Part print with two shaded views. Sizes in mm from the minimum x, y, z corner. A direction names the side the tool comes from. Round coordinates to 2 decimals unless told otherwise and drop trailing zeros. Loops run counter-clockwise (first coordinate to the right, second up) from the corner with the lowest first, then second, coordinate; pieces in that order, holes last. Notation, with made-up numbers: (44, -25.5) - (79, -25.5) arc R26 ccw to (79, -5.5) - close; hole circle Ø3 at (31, -8). An arc over 180 degrees is marked (long way). One line per question, with ' | ' between items.
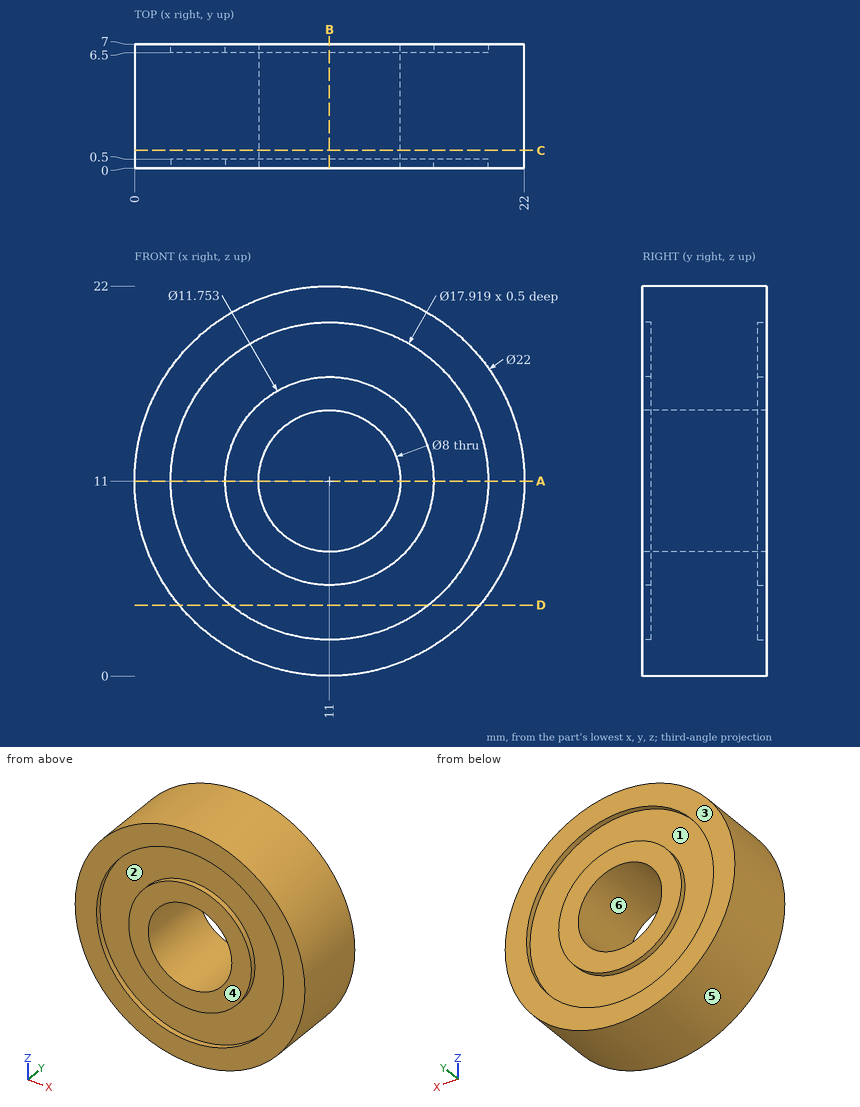
(1) Drop flat-ended pins along their axis: P1, Ø4, axis at x = 18, y = 2, coming from the +Z side; P2, Ø4, axis at x = 8, y = 1, coming from the +Z side; P3, Ø1, axis at y = 5.5, z = 12.5, coming from the -X side. Give the stop position or say it passes through.
Results found:
P1: stops at z = 20.8 | P2: stops at z = 21.95 | P3: stops at x = 0.05
(2) Cut at C-C, the plane y = 1. Write the cut outline in (x, z), then the cut area to 3 significant figures.
Results found:
outline: circle Ø22 at (11, 11); hole circle Ø8 at (11, 11) | area: 330 mm²
(3) Two-plate mould, pull along Z, no slides. Class the marked faces 4, 5 and 6: released by +Z, released by -Z, zero draft, split by the parting line, or undercut.
Results found:
face 4: zero draft | face 5: split by the parting line | face 6: undercut
(4) Probe L1, parallel to X at y = 6.95, z = 11; L2, parallel to X at y = 5.75, z = 11. List the from-to ranges inside material, lowest first.
Results found:
L1: x = 0 to 2.04, 5.12 to 7, 15 to 16.88, 19.96 to 22 | L2: x = 0 to 7, 15 to 22
(5) Cut at B-B, the plane x = 11. Write the cut outline in (y, z).
Results found:
outline: (0, 0) - (7, 0) - (7, 2.04) - (6.5, 2.04) - (6.5, 5.12) - (7, 5.12) - (7, 7) - (0, 7) - (0, 5.12) - (0.5, 5.12) - (0.5, 2.04) - (0, 2.04) - close; (0, 15) - (7, 15) - (7, 16.88) - (6.5, 16.88) - (6.5, 19.96) - (7, 19.96) - (7, 22) - (0, 22) - (0, 19.96) - (0.5, 19.96) - (0.5, 16.88) - (0, 16.88) - close
(6) Tool access for the marked faces 1, 2 and 3: list every direction of +Z, -Z, +X, -X, +Y, -Y with a clear straight run to the whole face (end or side of a thin tool).
Results found:
face 1: +Y | face 2: -Y | face 3: +Z, -Z, +X, -X, +Y
(7) Cut at A-A, the plane z = 11. Write the cut outline in (x, y).
Results found:
outline: (0, 0) - (2.04, 0) - (2.04, 0.5) - (5.12, 0.5) - (5.12, 0) - (7, 0) - (7, 7) - (5.12, 7) - (5.12, 6.5) - (2.04, 6.5) - (2.04, 7) - (0, 7) - close; (15, 0) - (16.88, 0) - (16.88, 0.5) - (19.96, 0.5) - (19.96, 0) - (22, 0) - (22, 7) - (19.96, 7) - (19.96, 6.5) - (16.88, 6.5) - (16.88, 7) - (15, 7) - close
(8) Cut at D-D, the plane z = 4. Write the cut outline in (x, y) (1 decimal).
Results found:
outline: (2.5, 0) - (5.4, 0) - (5.4, 0.5) - (16.6, 0.5) - (16.6, 0) - (19.5, 0) - (19.5, 7) - (16.6, 7) - (16.6, 6.5) - (5.4, 6.5) - (5.4, 7) - (2.5, 7) - close
